from build123d import *

# Parameters (mm, degrees)
F0_W = 12.7
F0_H = 12.7
F2_R = 6.34999


# Not quite as in the source:
# - a fillet or chamfer is up to 0.001 mm smaller than in the source, because OpenCascade refuses the exact size


with BuildPart() as f1:
    # F0 (on Front) → F1 (revolve)
    with BuildSketch(Plane.XZ):
        with Locations((19.05, 6.35)):
            Rectangle(F0_W, F0_H)
    revolve(axis=Axis((0, 0, 6.35), (0, 0, 1)))

    # F2 (radius 6.35 in the source; OpenCascade refuses exactly that, so slightly less here)
    f2_edges = [f1.edges().sort_by_distance(p)[0] for p in [
        (-25.4, 0, 12.7),
        (-12.7, 0, 12.7),
        (-12.7, 0, 0),
        (-25.4, 0, 0),
    ]]
    fillet(f2_edges, radius=F2_R)


solid = f1.part
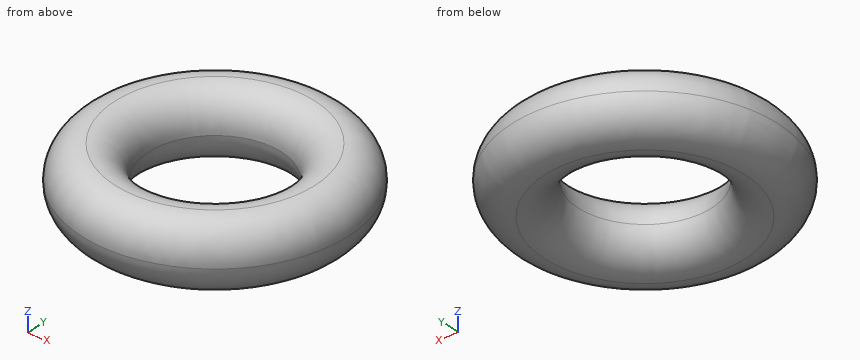
Here's how the part is built. I have some questions about the finished solid (model axes, mm). Coordinates: 2 decimals unless noted, no trailing zeros. Write each loop counter-clockwise with the first axis right and the second up, starting at its lowest first coordinate (ties: lowest second). Pieces come first, ordered by that corner, then holes.
1) If we section it at C-C (z = 9.25): List the corners of the cut face in (x, y) for me, plus the area to 3 significant figures.
Filled in:
outline: circle Ø49.4 at (0, 0); hole circle Ø26.8 at (0, 0)
area: 1,350 mm2
2) If I drill on line 1 (Y direction, x = 0, z = 6.45); line 2 (X direction, y = -1.5, z = 9); line 3 (X direction, y = 7.5, z = 10.25), over which ranges is the centre line in solid material (lowest first)?
Filled in:
line 1: y = -25.4 to -12.7, 12.7 to 25.4
line 2: x = -24.78 to -13.19, 13.19 to 24.78
line 3: x = -22.86 to -11.87, 11.87 to 22.86
3) I'm going to push flat-ended pins straight in: pin 1 (6 mm diameter, centred on y = -7.5, z = 4, fed in from -X); pin 2 (1.5 mm diameter, centred on y = -6.5, z = 10, fed in from -X); pin 3 (4 mm diameter, centred on x = -6, z = 9, fed in from +Y). Where does each tip first touch, or does it pass through?
Filled in:
pin 1: stops at x = -24.87
pin 2: stops at x = -23.87
pin 3: stops at y = 24.86
4) If we section it at D-D (z = 3.25): List the corners of the cut face in (x, y) for me.
Filled in:
outline: circle Ø49.18 at (0, 0); hole circle Ø27.02 at (0, 0)
